```python
from build123d import *

# Parameters (mm, degrees)
BOSS_EXTRUDE1_DEPTH = 736.6


with BuildPart() as part:
    # Sketch1 → Boss-Extrude1 (new body)
    with BuildSketch(Plane.XY):
        with BuildLine():
            Line((540.766, 306.324), (540.766, 528.32))
            Line((540.766, 528.32), (631.698, 528.32))
            Line((631.698, 528.32), (631.698, 550.164))
            Line((631.698, 550.164), (631.698, 746.76))
            Line((631.698, 746.76), (0, 746.76))
            Line((0, 746.76), (0, 604.52))
            Line((0, 604.52), (-35.56, 604.52))
            ThreePointArc((-35.56, 604.52), (-135.060085104, 537.524952941), (-15.461288674, 528.32))
            Line((-15.461288674, 528.32), (0, 528.32))
            Line((0, 528.32), (0, 0))
            Line((0, 0), (-25.4, 0))
            Line((-25.4, 0), (-25.4, -121.158))
            Line((-25.4, -121.158), (50.8, -121.158))
            Line((50.8, -121.158), (50.8, 0))
            Line((50.8, 0), (500.126, 0))
            Line((500.126, 0), (500.126, -121.158))
            Line((500.126, -121.158), (591.566, -121.158))
            Line((591.566, -121.158), (591.566, 0))
            Line((591.566, 0), (540.766, 0))
            Line((540.766, 0), (540.766, 264.16))
            Line((540.766, 264.16), (594.106, 264.16))
            Line((594.106, 264.16), (594.106, 2.032))
            Line((594.106, 2.032), (642.704381111, 2.032))
            Line((642.704381111, 2.032), (642.704381111, 264.16))
            Line((642.704381111, 264.16), (812.8, 264.16))
            Line((812.8, 264.16), (812.8, 306.324))
            Line((812.8, 306.324), (540.766, 306.324))
        make_face()
    extrude(amount=BOSS_EXTRUDE1_DEPTH)


solid = part.part
```
Source: CAD feature listing. Evaluate the final solid. Frame: model axes, mm. A direction names the side the tool comes from. Give positions to 0.01 mm unless a question says otherwise; leave off trailing zeros. Loops run counter-clockwise (first coordinate to the right, second up) from the corner with the lowest first, then second, coordinate; pieces in that order, holes last. Notation, with made-up numbers: (-2.75, 23) - (19.25, 23) arc R14 ccw to (19.25, 43) - close; hole circle Ø8 at (-37, 17). An arc over 180 degrees is marked (long way). Use CSV: the item, a comma, the result in double quotes. Start each with the question number.
1. Reachability of faces 1 (the flat face through (500.126, -60, 363)), 2 (the flat face through (540.766, 130, 363)), 3 (the flat face through (540.766, 416, 363)), 4 (the flat face through (642.704, 131, 363)) from +Z, -Z, +X, -X, +Y, -Y: full face, straight path, thin tool, end or side. Return the list, or none.
2. Ray query, L1, parallel to X at y = -42.5, z = 458.5; L2, parallel to X at y = 159.5, z = 264; L3, parallel to Y at x = 412.5, z = 241.5. Return the intervals inside material, ascending.
3. Pin query (flat end, axial travel): pin 1 (10 mm diameter, centred on x = -25.5, z = 648, fed in from +Y); pin 2 (1.5 mm diameter, centred on x = 344.5, y = 130, fed in from -Z); pin 3 (1 mm diameter, centred on x = 712.5, z = 389.5, fed in from +Y); pin 4 (24.5 mm diameter, centred on x = 618.5, z = 395.5, fed in from -Y). Return the tip coordinate at first contact, or that it passes through.
4. Section A-A (y = 87). Output: boundary loops of the cut face in (x, z).
5. Section B-B (x = 553). Output: boundary loops of the cut face in (y, z), then the cut area to 3 significant figures.
6. Draft query along Y for faces 5 (the flat face through (-18, 604.52, 363)), 6 (the flat face through (679, 306.324, 363)), 7 (the flat face through (0, 677, 363)). Return one class per face: +Y half, -Y half, draft (parallel to the pull), parting line (faces both ways), or undercut.
7. Section D-D (x = 152). Output: boundary loops of the cut face in (y, z).
8. Section C-C (z = 248.5). Output: boundary loops of the cut face in (x, y).
Response:
1,face 1,"+Z, -Z, -Y"
1,face 2,"+Z, -Z"
1,face 3,"+Z, -Z, +X"
1,face 4,"+Z, -Z, +X, -Y"
2,L1,"-25.4 to 50.8, 500.13 to 591.57"
2,L2,"0 to 540.77, 594.11 to 642.7"
2,L3,"0 to 746.76"
3,pin 1,"y = 604.52"
3,pin 2,"z = 0"
3,pin 3,"y = 306.32"
3,pin 4,"y = 2.03"
4,outline,"(0, 0) - (540.77, 0) - (540.77, 736.6) - (0, 736.6) - close; (594.11, 0) - (642.7, 0) - (642.7, 736.6) - (594.11, 736.6) - close"
5,outline,"(-121.16, 0) - (0, 0) - (0, 736.6) - (-121.16, 736.6) - close; (264.16, 0) - (306.32, 0) - (306.32, 736.6) - (264.16, 736.6) - close; (528.32, 0) - (746.76, 0) - (746.76, 736.6) - (528.32, 736.6) - close"
5,area,"281,000 mm²"
6,face 5,"+Y half"
6,face 6,"undercut"
6,face 7,"draft"
7,outline,"(0, 0) - (746.76, 0) - (746.76, 736.6) - (0, 736.6) - close"
8,outline,"(-35.56, 604.52) arc R63.5 ccw (long way) to (-15.46, 528.32) - (0, 528.32) - (0, 0) - (-25.4, 0) - (-25.4, -121.16) - (50.8, -121.16) - (50.8, 0) - (500.13, 0) - (500.13, -121.16) - (591.57, -121.16) - (591.57, 0) - (540.77, 0) - (540.77, 264.16) - (594.11, 264.16) - (594.11, 2.03) - (642.7, 2.03) - (642.7, 264.16) - (812.8, 264.16) - (812.8, 306.32) - (540.77, 306.32) - (540.77, 528.32) - (631.7, 528.32) - (631.7, 746.76) - (0, 746.76) - (0, 604.52) - close"
